Geometry: final body of the model. Coordinates: model frame, mm. A direction names the side the tool comes from. Give positions to 0.01 mm unless a question says otherwise; leave off trailing zeros. Write each loop counter-clockwise with the first axis right and the second up, starting at its lowest first coordinate (ties: lowest second). Pieces come first, ordered by that corner, then holes. Notation, with made-up numbers: M -7,86 L -2,86 A30 ccw -2,116 Z; hole C -1,54 d11. An arc over 180 degrees is marked long. Use a Markdown table: item, result. Add a question column.
(1) Cut plane D-D (x = 35). Output: boundary loops of the cut face in (y, z), plus the area to 3 significant figures.
(2) Cut plane B-B (x = -30). Output: boundary loops of the cut face in (y, z), plus the area to 3 significant figures.
(3) Cut plane A-A (y = 34). Output: boundary loops of the cut face in (x, z).
(4) Cut plane C-C (z = -5.5). Output: boundary loops of the cut face in (x, y), plus the area to 3 significant figures.
(5) Pin query (flat end, axial travel): pin 1 Ø2 at (x, z) = (-7.5, -32) entering from +Y; pin 2 Ø6 at (x, z) = (16.5, -40) entering from -Y. Return the tip coordinate at first contact, or that it passes through.
(6) Reachability of faces 1 (the flat face through (-14, 58, 35)), 2 (the flat face through (-40, 69, -35)) from +Z, -Z, +X, -X, +Y, -Y: full face, straight path, thin tool, end or side. Return the list, or none.
(7) Material intervals for L1, parallel to Z at x = 100, y = 135; L2, parallel to Y at x = 17.5, z = -31.5; L3, parallel to X at y = 41.5, z = -46, sorted ascending.
```python
from build123d import *

# Parameters (mm, degrees)
F0_W     = 260
F0_H     = 260
F1_DEPTH = 35
F2_SIZE  = 3
F3_R     = 60
F4_DEPTH = 15
F5_R     = 59.7511721788
F5_R_2   = 30
F6_DEPTH = 20
F7_DEPTH = 7
F8_DEPTH = 33.17


with BuildPart() as f1:
    # F0 (on Top) → F1 (new body)
    with BuildSketch(Plane.XY):
        with Locations((-12.1650248766, 56.3838380575)):
            Rectangle(F0_W, F0_H)
    extrude(amount=F1_DEPTH)

    # F2
    f2_edges = [f1.edges().sort_by_distance(p)[0] for p in [
        (117.834975, -73.616162, 17.5),
        (117.834975, 186.383838, 17.5),
        (-142.165025, 186.383838, 17.5),
        (-142.165025, -73.616162, 17.5),
    ]]
    chamfer(f2_edges, length=F2_SIZE)

    # F3 (on face) → F4 (join)
    with BuildSketch(Plane(origin=(0, 0, 0), x_dir=(1, 0, 0), z_dir=(0, 0, -1))):
        with Locations((-12.1650248766, -56.3838380575)):
            Circle(F3_R)
    extrude(amount=F4_DEPTH)

    # F5 (on face) → F6 (join)
    with BuildSketch(Plane(origin=(0, 0, -15), x_dir=(1, 0, 0), z_dir=(0, 0, -1))):
        with Locations((-12.1650248766, -56.3838380575)):
            Circle(F5_R)
        with Locations((-12.1650248766, -56.3838380575)):
            Circle(F5_R_2, mode=Mode.SUBTRACT)
    extrude(amount=F6_DEPTH)

    # F7 (add): a face of the model
    f7_faces = [f1.faces().sort_by_distance(p)[0] for p in [
        (-12.1650248766, 56.3838380575, -15),
    ]]
    extrude(f7_faces, amount=F7_DEPTH)

    # F8 (add): a face of the model
    f8_faces = [f1.faces().sort_by_distance(p)[0] for p in [
        (-12.1650248766, 56.3838380575, -22),
    ]]
    extrude(f8_faces, amount=F8_DEPTH)


solid = f1.part
```
Answer list:
| question | item | result |
|---|---|---|
| 1 | outline | M -73.62,0 L 19.3,0 L 19.3,-15 L 19.7,-15 L 19.7,-35 L 93.07,-35 L 93.07,-15 L 93.47,-15 L 93.47,0 L 186.38,0 L 186.38,35 L -73.62,35 Z |
| 1 | area | 11,700 mm² |
| 2 | outline | M -73.62,0 L -0.9,0 L -0.9,-15 L -0.64,-15 L -0.64,-35 L 32.26,-35 L 32.26,-55.17 L 80.51,-55.17 L 80.51,-35 L 113.41,-35 L 113.41,-15 L 113.67,-15 L 113.67,0 L 186.38,0 L 186.38,35 L -73.62,35 Z |
| 2 | area | 14,100 mm² |
| 3 | outline | M -142.17,0 L -67.83,0 L -67.83,-15 L -67.57,-15 L -67.57,-35 L -32.14,-35 L -32.14,-55.17 L 7.81,-55.17 L 7.81,-35 L 43.24,-35 L 43.24,-15 L 43.5,-15 L 43.5,0 L 117.83,0 L 117.83,35 L -142.17,35 Z |
| 4 | outline | C -12.17,56.38 d120 |
| 4 | area | 11,300 mm² |
| 5 | pin 1 | y = 116.02 |
| 5 | pin 2 | y = 40.85 |
| 6 | face 1 | +Z, +X, -X, +Y, -Y |
| 6 | face 2 | -Z |
| 7 | L1 | 0 to 35 |
| 7 | L2 | 4.52 to 108.25 |
| 7 | L3 | -38.21 to 13.88 |
